Source: CAD feature listing. Evaluate the final solid. Frame: model axes, mm. Face numbers are marked on the shaded views. A direction names the side the tool comes from. Give positions to 0.01 mm unless a question says otherwise; leave off trailing zeros. Write each loop counter-clockwise with the first axis right and the second up, starting at its lowest first coordinate (ties: lowest second). Pieces come first, ordered by that corner, then holes. Notation, with made-up numbers: (81, 72) - (123, 72) arc R15 ccw to (123, 78) - close; hole circle Ø5 at (66.25, -21.5). An arc over 180 degrees is marked (long way). One line per question, with ' | ' between items. Start each with the question number.
(1) Section D-D, the plane x = 130.5. Return loops of the section in (y, z).
(2) Section B-B, the plane x = 93.5. Return loops of the section in (y, z), plus the area to 3 significant figures.
(3) Ray query, line 1 (X direction, y = 3.5, z = 7.25); line 2 (Y direction, x = 112, z = -2.75); line 3 (Z direction, x = 121, y = 15.75). Return the intervals inside material, ascending. Write a range as [from, to].
(4) Pin query (flat end, axial travel): pin 1 (12 mm diameter, centred on x = 105, z = 8, fed in from -Y); pin 2 (1 mm diameter, centred on x = 103, y = 10.5, fed in from +Z); pin 3 (6.5 mm diameter, centred on x = 119.5, z = -0.5, fed in from +Y); pin 4 (9 mm diameter, centred on y = 4.5, z = -4, fed in from +X). Return the tip coordinate at first contact, or that it passes through.
(5) Section A-A, the plane y = 8. Return loops of the section in (x, z), plus the area to 3 significant figures.
(6) Draft query along Z for the marked faces 4 and 5. Return one class per face: +Z half, -Z half, draft (parallel to the pull), parting line (faces both ways), or undercut.
(7) Section C-C, the plane z = 0.25. Return loops of the section in (x, y), plus the area to 3 significant figures.
(8) Access query for the marked faces 1, 2 and 3. Directions: +Z, -Z, +X, -X, +Y, -Y. A direction counts if a zero-diameter tool reaches every point of the face in a straight line with its end or side. Return the directions, or none.
```python
from build123d import *

# Parameters (mm, degrees)
BOSS_EXTRUDE1_DEPTH     = 17.5
SKETCH2_W               = 252
SKETCH2_H               = 14.5
CUT_EXTRUDE1_DEPTH      = 15.5
SKETCH3_R               = 13
CUT_EXTRUDE2_DEPTH      = 15.5
CUT_EXTRUDE3_REACH      = 264.265
CUT_EXTRUDE3_END_RADIUS = 13
SKETCH5_W               = 252
SKETCH5_H               = 1
BOSS_EXTRUDE2_DEPTH     = 2
SKETCH6_R               = 1
CUT_EXTRUDE4_DEPTH      = 2
CUT_EXTRUDE9_DEPTH      = 278.209870862


with BuildPart() as part:
    # Sketch1 → Boss-Extrude1 (new body)
    with BuildSketch(Plane(origin=(0, 0, 0), x_dir=(1, 0, 0), z_dir=(0, 1, 0))):
        with BuildLine():
            Line((0.323033708, 14.996521237), (267.19920412, 9.247854763))
            ThreePointArc((267.19920412, 9.247854763), (276.25, 0), (267.19920412, -9.247854763))
            Line((267.19920412, -9.247854763), (0.323033708, -14.996521237))
            ThreePointArc((0.323033708, -14.996521237), (-15, 0), (0.323033708, 14.996521237))
        make_face()
    extrude(amount=BOSS_EXTRUDE1_DEPTH)

    # Sketch2 → Cut-Extrude1 (cut)
    with BuildSketch(Plane(origin=(0, 17.5, 0), x_dir=(1, 0, 0), z_dir=(0, 1, 0))):
        with Locations((141, 0)):
            Rectangle(SKETCH2_W, SKETCH2_H)
    extrude(amount=-CUT_EXTRUDE1_DEPTH, mode=Mode.SUBTRACT)

    # Sketch3 → Cut-Extrude2 (cut)
    with BuildSketch(Plane(origin=(0, 17.5, 0), x_dir=(1, 0, 0), z_dir=(0, 1, 0))):
        with Locations(Location((0, 0, 0), (0, 0, 270))):
            Circle(SKETCH3_R)
    extrude(amount=-CUT_EXTRUDE2_DEPTH, mode=Mode.SUBTRACT)

    # Cut-Extrude3: up to this cylinder (the profile starts outside it)
    cut_extrude3_end = Plane(origin=(0, 8.125709, 0), z_dir=(0, 1, 0)) * Cylinder(CUT_EXTRUDE3_END_RADIUS, 555.53, mode=Mode.PRIVATE)
    # Sketch4 → Cut-Extrude3 (cut, up to the surface)
    with BuildSketch(Plane(origin=(15, 0, 0), x_dir=(0, 0, -1), z_dir=(1, 0, 0)), mode=Mode.PRIVATE) as cut_extrude3_sk1:
        with BuildLine():
            Line((-7.25, 2), (7.25, 2))
            Line((7.25, 2), (7.25, 8.5))
            ThreePointArc((7.25, 8.5), (5.199747468, 13.449747468), (0.25, 15.5))
            Line((0.25, 15.5), (-0.25, 15.5))
            ThreePointArc((-0.25, 15.5), (-5.199747468, 13.449747468), (-7.25, 8.5))
            Line((-7.25, 8.5), (-7.25, 2))
        make_face()
    cut_extrude3_tool1 = extrude(cut_extrude3_sk1.sketch, amount=-CUT_EXTRUDE3_REACH, mode=Mode.PRIVATE) - cut_extrude3_end
    add(cut_extrude3_tool1.solids().sort_by_distance((15, 8.125709, 0))[0], mode=Mode.SUBTRACT)

    # Sketch5 → Boss-Extrude2 (add)
    with BuildSketch(Plane(origin=(0, 2, 0), x_dir=(1, 0, 0), z_dir=(0, 1, 0))):
        with Locations((141, 6.75)):
            Rectangle(SKETCH5_W, SKETCH5_H)
        with Locations((141, -6.75)):
            Rectangle(SKETCH5_W, SKETCH5_H)
    extrude(amount=BOSS_EXTRUDE2_DEPTH)

    # Sketch6 → Cut-Extrude4 (cut)
    with BuildSketch(Plane(origin=(0, 2, 0), x_dir=(1, 0, 0), z_dir=(0, 1, 0))):
        with Locations(Location((-5.25, 9.09326674, 0), (0, 0, 270))):
            Circle(SKETCH6_R)
        with Locations(Location((-10.5, 0, 0), (0, 0, 270))):
            Circle(SKETCH6_R)
        with Locations(Location((5.25, 9.09326674, 0), (0, 0, 270))):
            Circle(SKETCH6_R)
        with Locations(Location((10.5, 0, 0), (0, 0, 270))):
            Circle(SKETCH6_R)
        with Locations(Location((5.25, -9.09326674, 0), (0, 0, 270))):
            Circle(SKETCH6_R)
        with Locations(Location((-5.25, -9.09326674, 0), (0, 0, 270))):
            Circle(SKETCH6_R)
        Polygon((0, -10), (8.660254038, -5), (8.660254038, 5), (0, 10), (-8.660254038, 5), (-8.660254038, -5), align=None)
    extrude(amount=-CUT_EXTRUDE4_DEPTH, mode=Mode.SUBTRACT)

    # Sketch14 → Cut-Extrude9 (cut, through all)
    with BuildSketch(Plane(origin=(0, 0, 0), x_dir=(1, 0, 0), z_dir=(0, 1, 0))):
        Polygon((88.5, 9.35), (78.6, 9.35), (78.6, 35), (78.4, 35), (78.4, 9.15), (88.3, 9.15), (88.3, -9.15), (78.4, -9.15), (78.4, -35), (78.6, -35), (78.6, -9.35), (88.5, -9.35), align=None)
        Polygon((172.7, 9.15), (182.6, 9.15), (182.6, 35), (182.4, 35), (182.4, 9.35), (172.5, 9.35), (172.5, 9.25), (172.5, -9.35), (182.4, -9.35), (182.4, -35), (182.6, -35), (182.6, -9.15), (172.7, -9.15), align=None)
    extrude(amount=CUT_EXTRUDE9_DEPTH, mode=Mode.SUBTRACT)


with BuildPart() as cut_extrude9_kept_piece:
    # of the separate pieces the step leaves, the one the design keeps (cut_extrude9_pieces_kept)
    add(part.part.solids().sort_by_distance((182.4, 0, 11.074478478))[0])


solid = cut_extrude9_kept_piece.part
```
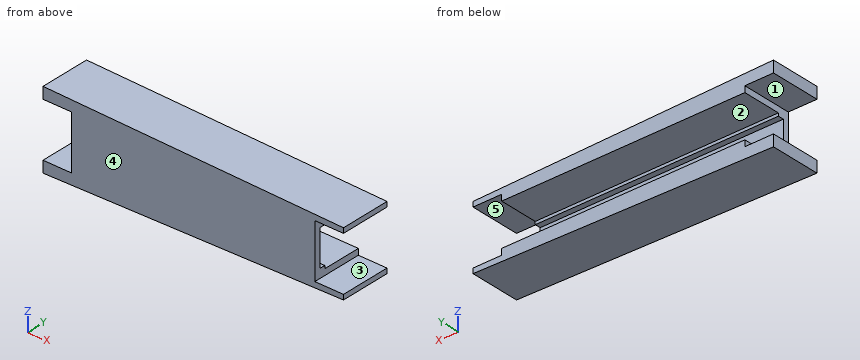
Check sheet entries:
1) outline: (0, -12.19) - (17.5, -12.19) - (17.5, -7.25) - (4, -7.25) - (4, -6.25) - (2, -6.25) - (2, 6.25) - (4, 6.25) - (4, 7.25) - (17.5, 7.25) - (17.5, 12.19) - (0, 12.19) - close
2) outline: (0, -12.99) - (17.5, -12.99) - (17.5, -7.25) - (4, -7.25) - (4, -6.25) - (2, -6.25) - (2, 6.25) - (4, 6.25) - (4, 7.25) - (17.5, 7.25) - (17.5, 12.99) - (0, 12.99) - close | area: 234 mm²
3) line 1: [88.5, 172.5] | line 2: [0, 2] | line 3: [-12.4, -7.25], [7.25, 12.4]
4) pin 1: y = 0 | pin 2: z = 12.8 | pin 3: y = 2 | pin 4: x = 172.5
5) outline: (78.6, -13.31) - (182.4, -11.07) - (182.4, -9.35) - (172.5, -9.35) - (172.5, -7.25) - (88.5, -7.25) - (88.5, -9.35) - (78.6, -9.35) - close; (78.6, 9.35) - (88.5, 9.35) - (88.5, 7.25) - (172.5, 7.25) - (172.5, 9.35) - (182.4, 9.35) - (182.4, 11.07) - (78.6, 13.31) - close | area: 943 mm²
6) face 4: draft | face 5: undercut
7) outline: (88.5, 0) - (172.5, 0) - (172.5, 2) - (88.5, 2) - close | area: 168 mm²
8) face 1: -X, +Y, -Y | face 2: +X, -X, +Y | face 3: +X, +Y, -Y
